```python
from build123d import *

# Parameters (mm, degrees)
F0_W     = 60.5
F0_H     = 4
F1_DEPTH = 10
F2_R     = 2.75
F3_DEPTH = 31.7
F4_SIZE  = 3
F5_W     = 29.333754
F5_H     = 4
F6_DEPTH = 1.5
F8_DEPTH = 5


with BuildPart() as f1:
    # F0 (on Right) → F1 (new body)
    with BuildSketch(Plane.YZ):
        Polygon((0, 25), (0, 0), (10, 0), (10, 4), (10, 25), align=None)
        with Locations((40.25, 2)):
            Rectangle(F0_W, F0_H)
    extrude(amount=F1_DEPTH)

    # F2 (on face) → F3 (cut)
    with BuildSketch(Plane.XY.offset(4)):
        with Locations((6, 53.3)):
            Circle(F2_R)
        with Locations((6, 63.5)):
            Circle(F2_R)
    extrude(amount=-F3_DEPTH, mode=Mode.SUBTRACT)

    # F4
    f4_edges = [f1.edges().sort_by_distance(p)[0] for p in [
        (0, 0, 12.5),
        (0, 10, 14.5),
    ]]
    chamfer(f4_edges, length=F4_SIZE)

    # F5 (on face) → F6 (cut)
    with BuildSketch(Plane(origin=(0, 0, 0), x_dir=(0, -1, 0), z_dir=(-1, 0, 0))):
        with Locations((-55.833123, 2)):
            Rectangle(F5_W, F5_H)
    extrude(amount=-F6_DEPTH, mode=Mode.SUBTRACT)

    # F7 (on face) → F8 (join)
    with BuildSketch(Plane.YZ.offset(10)):
        Polygon((25, 4), (10, 20), (10, 4), align=None)
    extrude(amount=-F8_DEPTH)


solid = f1.part
```
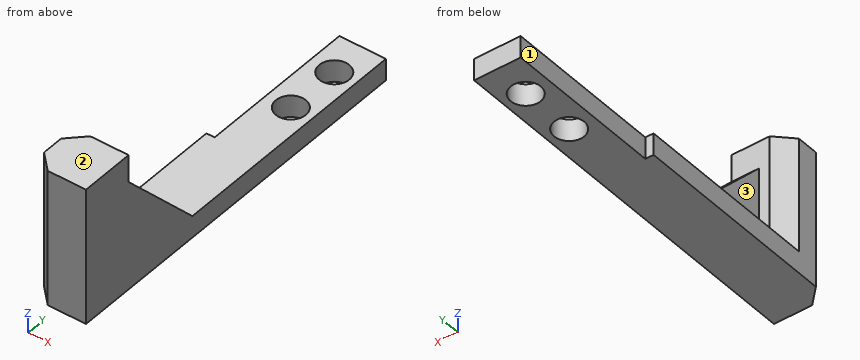
Can you work these out from the model? Positions are in its coordinate system, mm. Face numbers are marked on the shaded views. A direction names the side the tool comes from. Round coordinates to 2 decimals unless told otherwise and drop trailing zeros. Loops run counter-clockwise (first coordinate to the right, second up) from the corner with the lowest first, then second, coordinate; pieces in that order, holes last. Notation, with made-up numbers: M 27,23.5 L 38,23.5 A15 ccw 38,42.5 Z; hole C 37,-32.75 d8. An arc over 180 degrees is marked long. Write item = value, one per line. Start each with the question number.
(1) Which directions (+Z, -Z, +X, -X, +Y, -Y) give clear straight access to the entire face, cutting with the end or side of a thin tool? Please do the marked faces 1, 2 and 3.
(2) Suppose I cut it at C-C on y = 53.3. Write out the boundary of the cut face in (x, z).
(3) Suppose I cut it at B-B on z = 3.25. Write out the boundary of the cut face in (x, y), plus the area to 3 significant figures.
(4) I need wall thicknesses on line 1 along Y through (x, z) = (6, 1.85); line 2 along Y through (x, z) = (6.5, 24); line 3 along Z through (x, y) = (3, 45). Which ranges of each line are inside material? Lowest first, please.
(5) I'm going to push flat-ended pins straight in: P1, Ø4.5, axis at y = 49.5, z = 2.5, coming from the -X side; P2, Ø5.5, axis at x = 6, z = 10.5, coming from the +Y side. Where does each tip first touch, or does it pass through?
(6) Suppose I cut it at A-A on x = 6. Write out the boundary of the cut face in (y, z), plus the area to 3 significant figures.
(7) Suppose I cut it at D-D on y = 20.5. Write out the boundary of the cut face in (x, z).
Answer block:
q1.face_1 = +Z, -Z, -X, +Y
q1.face_2 = +Z, +X, -X, +Y, -Y
q1.face_3 = +Z, -X, +Y
q2.outline = M 1.5,0 L 3.25,0 L 3.25,4 L 1.5,4 Z; M 8.75,0 L 10,0 L 10,4 L 8.75,4 Z
q3.outline = M 0,3 L 3,0 L 10,0 L 10,70.5 L 1.5,70.5 L 1.5,41.17 L 0,41.17 Z; hole C 6,53.3 d5.5; hole C 6,63.5 d5.5
q3.area = 609 mm²
q4.line_1 = 0 to 50.55, 56.05 to 60.75, 66.25 to 70.5
q4.line_2 = 0 to 10
q4.line_3 = 0 to 4
q5.P1 = 1.5
q5.P2 = 21.48
q6.outline = M 0,0 L 50.55,0 L 50.55,4 L 25,4 L 10,20 L 10,25 L 0,25 Z; M 56.05,0 L 60.75,0 L 60.75,4 L 56.05,4 Z; M 66.25,0 L 70.5,0 L 70.5,4 L 66.25,4 Z
q6.area = 568 mm²
q7.outline = M 0,0 L 10,0 L 10,8.8 L 5,8.8 L 5,4 L 0,4 Z
